from build123d import *

# Parameters (mm, degrees)
SKETCH1_R           = 3
BOSS_EXTRUDE1_DEPTH = 31.5
SKETCH4_R           = 2
SKETCH9_R           = 3
BOSS_EXTRUDE2_DEPTH = 31.5


with BuildPart() as part:
    # Sketch1 → Boss-Extrude1 (new body)
    with BuildSketch(Plane.XY):
        Circle(SKETCH1_R)
    extrude(amount=BOSS_EXTRUDE1_DEPTH)

    # Sweep1: sweep along a path in Sketch5
    with BuildLine(Plane(origin=(0, 0, 0), x_dir=(0, 0, -1), z_dir=(1, 0, 0))) as sweep1_path:
        ThreePointArc((0, 0), (3.535533906, 1.464466094), (5, 5))
    # Sketch4 → Sweep1 (sweep)
    with BuildSketch(Plane(origin=(0, 0, 0), x_dir=(-1, 0, 0), z_dir=(0, 0, -1))):
        Circle(SKETCH4_R)
    sweep(path=sweep1_path.line)

    # Sketch9 → Boss-Extrude2 (add)
    with BuildSketch(Plane(origin=(0, 5, 0), x_dir=(1, 0, 0), z_dir=(0, 1, 0))):
        with Locations(Location((0, 5, 0), (0, 0, 270))):
            Circle(SKETCH9_R)
    extrude(amount=BOSS_EXTRUDE2_DEPTH)


solid = part.part
The model under review builds one solid part; all positions refer to its coordinate system, in mm. A direction names the side the tool comes from. Give positions to 0.01 mm unless a question says otherwise; leave off trailing zeros. Order: outer loops, then holes, each group sorted by start corner. A loop starts at its lowest first (then second) coordinate and runs counter-clockwise, first axis right, second up. Notation, with made-up numbers: M 71.25,40.25 L 105.25,40.25 A24 cw 105.25,52.25 Z; hole C 15.5,-17 d1. An arc over 180 degrees is marked long. One line per question, with ' | ' between items. Start each with the question number.
1) Clearance check with flat-ended pins moving along their axes: P1, Ø1.8, axis at x = 0, z = -3.5, coming from the -Y side; P2, Ø1, axis at x = -1.5, z = -2.5, coming from the -Y side; P3, Ø3, axis at x = -1, z = 21, coming from the -Y side; P4, Ø6, axis at y = 20, z = -1.5, coming from the -X side. State where each tip first meets the part, or that it passes through.
2) Mouldability with a two-part tool opening along Z and no side actions: class faces 3 (the face through (0.9, 20.53, -2.14)), 4 (the face through (-3, 0, 16)), 5 (the face through (1, -2, 0)) as pulls with the +Z half, pulls with the -Z half, needs draft (parallel to the pull), parting line crosses it, or undercut.
3) Consider section C-C, the plane y = 25. Give the boundary of the cut face in (x, z), then the cut area to 3 significant figures.
4) Consider section B-B, the plane z = 5. Give the boundary of the cut face in (x, y).
5) Consider section A-A, the plane x = 0. Give the boundary of the cut face in (y, z).
6) Wall thickness on L1, parallel to Y at x = 0.15, z = 16.5; L2, parallel to Z at x = -2.3, y = 0; L3, parallel to Y at x = -2.4, z = -5.5: over which ranges is each line inside the solid? List them lowest first. Write a range as from..to.
7) For faces 1 (the face through (-2, 5, -4)), 2 (the face through (0, 0, 31.5)), list the 3-axis set-ups (+Z, -Z, +X, -X, +Y, -Y) from which the entire face can be reached by the end or side of a thin tool; tool diameter is ignored.
Found:
1) P1: stops at y = -1.5 | P2: stops at y = -1.3 | P3: stops at y = -3 | P4: stops at x = -2.96
2) face 3: parting line crosses it | face 4: needs draft | face 5: undercut
3) outline: C 0,-5 d6 | area: 28.3 mm²
4) outline: C 0,0 d6
5) outline: M -3,0 L -2,0 A7 ccw 5,-7 L 5,-8 L 36.5,-8 L 36.5,-2 L 5,-2 L 5,-3 A3 cw 2,0 L 3,0 L 3,31.5 L -3,31.5 Z
6) L1: y = -3..3 | L2: z = 0..31.5 | L3: y = 5..36.5
7) face 1: none | face 2: +Z, +X, -X, +Y, -Y
